```python
from build123d import *

# Parameters (mm, degrees)
SKETCH_1_R          = 2
SKETCH_1_R_2        = 3.55
EXTRUDE_1_DEPTH     = 4
EXTRUDE_3_DEPTH     = 4
SKETCH_3_R          = 3.6
CUT_EXTRUDE_1_DEPTH = 1.4
SKETCH_7_R          = 2
CUT_EXTRUDE_2_DEPTH = 10
SKETCH_8_R          = 3.6
CUT_EXTRUDE_3_DEPTH = 1.3


with BuildPart() as part:
    # 草图1 → 凸台-拉伸1 (new body)
    with BuildSketch(Plane.XY):
        with BuildLine():
            Line((-180.694062755, -12.410089261), (126.305937245, -12.410089261))
            ThreePointArc((126.305937245, -12.410089261), (129.13436437, -11.238516386), (130.305937245, -8.410089261))
            Line((130.305937245, -8.410089261), (130.305937245, 7.71191214))
            Line((130.305937245, 7.71191214), (130.305937245, 17.589910739))
            Line((130.305937245, 17.589910739), (130.305937245, 39.589910739))
            ThreePointArc((130.305937245, 39.589910739), (129.13436437, 42.418337863), (126.305937245, 43.589910739))
            Line((126.305937245, 43.589910739), (-23.194062755, 43.589910739))
            ThreePointArc((-23.194062755, 43.589910739), (-26.022489879, 42.418337863), (-27.194062755, 39.589910739))
            Line((-27.194062755, 39.589910739), (-27.194062755, 27.589910739))
            ThreePointArc((-27.194062755, 27.589910739), (-30.122994943, 20.518842927), (-37.194062755, 17.589910739))
            Line((-37.194062755, 17.589910739), (-180.694062755, 17.589910739))
            ThreePointArc((-180.694062755, 17.589910739), (-183.522489879, 16.418337863), (-184.694062755, 13.589910739))
            Line((-184.694062755, 13.589910739), (-184.694062755, -8.410089261))
            ThreePointArc((-184.694062755, -8.410089261), (-183.522489879, -11.238516386), (-180.694062755, -12.410089261))
        make_face()
        with Locations((-127.194062755, -7.410089261)):
            Circle(SKETCH_1_R, mode=Mode.SUBTRACT)
        with Locations((-88.864062755, -7.410089261)):
            Circle(SKETCH_1_R, mode=Mode.SUBTRACT)
        with Locations((34.475937245, -7.410089261)):
            Circle(SKETCH_1_R, mode=Mode.SUBTRACT)
        with Locations((72.805937245, -7.410089261)):
            Circle(SKETCH_1_R, mode=Mode.SUBTRACT)
        with Locations((34.475937245, 38.589910739)):
            Circle(SKETCH_1_R, mode=Mode.SUBTRACT)
        with Locations((122.805937245, 31.589910739)):
            Circle(SKETCH_1_R_2, mode=Mode.SUBTRACT)
        with Locations((72.805937245, 38.589910739)):
            Circle(SKETCH_1_R, mode=Mode.SUBTRACT)
    extrude(amount=EXTRUDE_1_DEPTH)

    # 草图2 → 凸台-拉伸3 (add)
    with BuildSketch(Plane(origin=(0, 0, 0), x_dir=(-1, 0, 0), z_dir=(0, 0, -1))):
        with BuildLine():
            Line((53.194062755, 43.589910739), (23.194062755, 43.589910739))
            Line((23.194062755, 43.589910739), (23.194062755, 17.589910739))
            Line((23.194062755, 17.589910739), (57.194062755, 17.589910739))
            Line((57.194062755, 17.589910739), (61.194062755, 17.589910739))
            ThreePointArc((61.194062755, 17.589910739), (58.36563563, 18.761483614), (57.194062755, 21.589910739))
            Line((57.194062755, 21.589910739), (57.194062755, 39.589910739))
            ThreePointArc((57.194062755, 39.589910739), (56.022489879, 42.418337863), (53.194062755, 43.589910739))
        make_face()
    extrude(amount=-EXTRUDE_3_DEPTH)

    # 草图3 → 切除-拉伸1 (cut)
    with BuildSketch(Plane(origin=(0, 0, 0), x_dir=(-1, 0, 0), z_dir=(0, 0, -1))):
        with Locations((-72.805937245, 38.589910739)):
            Circle(SKETCH_3_R)
        with Locations((-34.475937245, 38.589910739)):
            Circle(SKETCH_3_R)
    extrude(amount=-CUT_EXTRUDE_1_DEPTH, mode=Mode.SUBTRACT)

    # 草图7 → 切除-拉伸2 (cut)
    with BuildSketch(Plane(origin=(0, 0, 0), x_dir=(-1, 0, 0), z_dir=(0, 0, -1))):
        with Locations((29.194062755, 32.589910739)):
            Circle(SKETCH_7_R)
    extrude(amount=-CUT_EXTRUDE_2_DEPTH, mode=Mode.SUBTRACT)

    # 草图8 → 切除-拉伸3 (cut)
    with BuildSketch(Plane.XY.offset(4)):
        with Locations((72.805937245, 38.589910739)):
            Circle(SKETCH_8_R)
        with Locations((34.475937245, 38.589910739)):
            Circle(SKETCH_8_R)
    extrude(amount=-CUT_EXTRUDE_3_DEPTH, mode=Mode.SUBTRACT)


solid = part.part
```
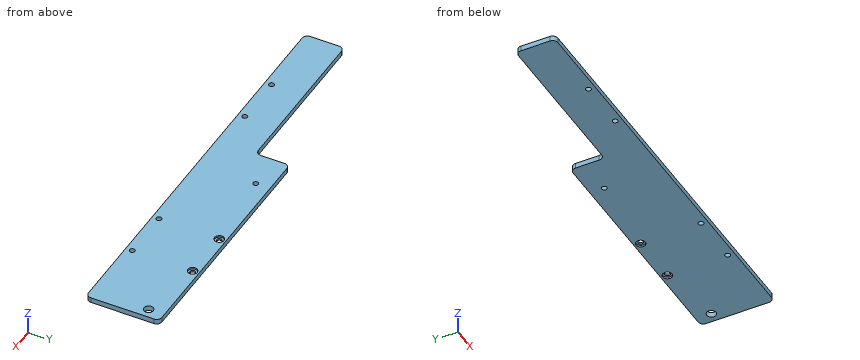
For this review, take the finished solid that the model builds, in its own axes (mm). Give positions to 0.01 mm unless a question says otherwise; leave off trailing zeros. Loops run counter-clockwise (first coordinate to the right, second up) from the corner with the lowest first, then second, coordinate; pieces in that order, holes last. Notation, with made-up numbers: M -30.75,48.5 L -0.75,48.5 A20 ccw -0.75,53.5 Z; hole C 68.25,81 d2. An arc over 180 degrees is marked long. One line per item, written item: value. Start each with the question number.
Q1. Add section A-A (x = -100.5). Give the boundary of the cut face in (y, z).
Q2. For L1, parallel to X at y = 41, z = 3.75; L2, parallel to Y at x = -165.5, z = 1.05; L3, parallel to X at y = 21.5, z = 2.4, list the stretches that pass through material, from the lowest coordinate up.
Q3. Clearance check with flat-ended pins moving along their axes: pin 1 Ø6.5 at (x, y) = (-88.86, -7.41) entering from +Z; pin 2 Ø6.5 at (x, y) = (34.48, 38.59) entering from +Z; pin 3 Ø3.5 at (x, y) = (-29.19, 32.59) entering from +Z; pin 4 Ø1 at (y, z) = (16.5, 2) entering from -X. State where each tip first meets the part, or that it passes through.
Reply:
1. outline: M -12.41,0 L 17.59,0 L 17.59,4 L -12.41,4 Z
2. L1: -56.94 to 31.8, 37.15 to 70.13, 75.48 to 130.05
2. L2: -12.41 to 17.59
2. L3: -57.2 to 130.31
3. pin 1: z = 4
3. pin 2: z = 2.7
3. pin 3: through
3. pin 4: x = -183.89
